Work out the finished part from the listing and answer in its coordinate system (mm). Coordinates: 2 decimals unless noted, no trailing zeros. Loops run counter-clockwise (first coordinate to the right, second up) from the corner with the lowest first, then second, coordinate; pieces in that order, holes last. Notation, with made-up numbers: (82, -27.75) -> (91, -27.75) arc R15 ccw to (91, -16.75) -> close; hole circle Ø1 at (-22, -8.75). An arc over 180 degrees is marked (long way). Use a Markdown table: item, result.
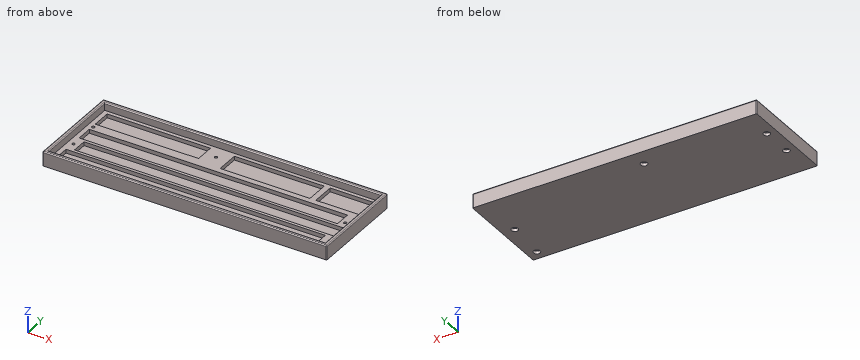
from build123d import *

# Parameters (mm, degrees)
SKETCH_W        = 297
SKETCH_H        = 102
PAD_DEPTH       = 15
SKETCH001_W     = 289
SKETCH001_H     = 94
POCKET_DEPTH    = 8
SKETCH002_W     = 271
SKETCH002_H     = 16
SKETCH002_W_2   = 272
SKETCH002_W_3   = 270
SKETCH002_H_2   = 17
SKETCH002_W_4   = 45.901761
SKETCH002_H_3   = 24
SKETCH002_W_5   = 94
SKETCH002_W_6   = 108
SKETCH002_H_4   = 20
POCKET001_DEPTH = 4
SKETCH003_R     = 1.51818
SKETCH003_R_2   = 1.523657
SKETCH003_R_3   = 1.522766
SKETCH003_R_4   = 1.49253
SKETCH003_R_5   = 1.485367
POCKET002_DEPTH = 15
SKETCH004_R     = 3.476644
SKETCH004_R_2   = 3.504577
SKETCH004_R_3   = 3.496918
SKETCH004_R_4   = 3.4664
SKETCH004_R_5   = 3.481812
POCKET003_DEPTH = 3
FILLET_R        = 1
FILLET001_R     = 1


with BuildPart() as part:
    # Sketch → Pad (new body)
    with BuildSketch(Plane.XY):
        with Locations((148.5, 51)):
            Rectangle(SKETCH_W, SKETCH_H)
    extrude(amount=PAD_DEPTH)

    # Sketch001 → Pocket (cut)
    with BuildSketch(Plane.XY.offset(15)):
        with Locations((148.5, 51)):
            Rectangle(SKETCH001_W, SKETCH001_H)
    extrude(amount=-POCKET_DEPTH, mode=Mode.SUBTRACT)

    # Sketch002 → Pocket001 (cut)
    with BuildSketch(Plane.XY.offset(7)):
        with Locations((144.5, 17)):
            Rectangle(SKETCH002_W, SKETCH002_H)
        with Locations((152, 36)):
            Rectangle(SKETCH002_W_2, SKETCH002_H)
        with Locations((144, 55.5)):
            Rectangle(SKETCH002_W_3, SKETCH002_H_2)
        with Locations((265.049119, 82)):
            Rectangle(SKETCH002_W_4, SKETCH002_H_3)
        with Locations((189, 82)):
            Rectangle(SKETCH002_W_5, SKETCH002_H_3)
        with Locations((63, 84)):
            Rectangle(SKETCH002_W_6, SKETCH002_H_4)
    extrude(amount=-POCKET001_DEPTH, mode=Mode.SUBTRACT)

    # Sketch003 → Pocket002 (cut)
    with BuildSketch(Plane.XY.offset(7)):
        with Locations((284, 52)):
            Circle(SKETCH003_R)
        with Locations((10, 36)):
            Circle(SKETCH003_R_2)
        with Locations((287, 10)):
            Circle(SKETCH003_R_3)
        with Locations((10, 69)):
            Circle(SKETCH003_R_4)
        with Locations((129, 84)):
            Circle(SKETCH003_R_5)
    extrude(amount=-POCKET002_DEPTH, mode=Mode.SUBTRACT)

    # Sketch004 → Pocket003 (cut)
    with BuildSketch(Plane(origin=(0, 0, 0), x_dir=(1, 0, 0), z_dir=(0, 0, -1))):
        with Locations((10, -36)):
            Circle(SKETCH004_R)
        with Locations((10, -69)):
            Circle(SKETCH004_R_2)
        with Locations((129, -84)):
            Circle(SKETCH004_R_3)
        with Locations((287, -10)):
            Circle(SKETCH004_R_4)
        with Locations((284, -52)):
            Circle(SKETCH004_R_5)
    extrude(amount=-POCKET003_DEPTH, mode=Mode.SUBTRACT)

    # Fillet
    fillet_edges = [part.edges().sort_by_distance(p)[0] for p in [
        (148.5, 102, 15),
        (297, 102, 7.5),
        (0, 102, 7.5),
        (148.5, 0, 15),
        (297, 0, 7.5),
        (0, 0, 7.5),
        (0, 51, 15),
        (297, 51, 15),
    ]]
    fillet(fillet_edges, radius=FILLET_R)

    # Fillet001
    fillet001_edges = [part.edges().sort_by_distance(p)[0] for p in [
        (148.5, 98, 15),
        (4, 51, 15),
        (148.5, 4, 15),
        (293, 51, 15),
    ]]
    fillet(fillet001_edges, radius=FILLET001_R)


solid = part.part
Q1. Section A-A on z = 11.5 is taken. Determine the outline of the cut face in (x, y), and give its area (3 significant figures).
Solved:
| item | result |
|---|---|
| outline | (0, 1) arc R1 ccw to (1, 0) -> (296, 0) arc R1 ccw to (297, 1) -> (297, 101) arc R1 ccw to (296, 102) -> (1, 102) arc R1 ccw to (0, 101) -> close; hole (4, 4) -> (293, 4) -> (293, 98) -> (4, 98) -> close |
| area | 3,130 mm² |
Q2. Section D-D on x = 95.5 is taken. Determine the outline of the cut face in (y, z), and give its area (3 significant figures).
Solved:
| item | result |
|---|---|
| outline | (0, 0) -> (102, 0) -> (102, 14) arc R1 ccw to (101, 15) -> (99, 15) arc R1 ccw to (98, 14) -> (98, 7) -> (94, 7) -> (94, 3) -> (74, 3) -> (74, 7) -> (64, 7) -> (64, 3) -> (47, 3) -> (47, 7) -> (44, 7) -> (44, 3) -> (28, 3) -> (28, 7) -> (25, 7) -> (25, 3) -> (9, 3) -> (9, 7) -> (4, 7) -> (4, 14) arc R1 ccw to (3, 15) -> (1, 15) arc R1 ccw to (0, 14) -> close |
| area | 501 mm² |
Q3. Section B-B on x = 201 is taken. Determine the outline of the cut face in (y, z), and give its area (3 significant figures).
Solved:
| item | result |
|---|---|
| outline | (0, 0) -> (102, 0) -> (102, 14) arc R1 ccw to (101, 15) -> (99, 15) arc R1 ccw to (98, 14) -> (98, 7) -> (94, 7) -> (94, 3) -> (70, 3) -> (70, 7) -> (64, 7) -> (64, 3) -> (47, 3) -> (47, 7) -> (44, 7) -> (44, 3) -> (28, 3) -> (28, 7) -> (25, 7) -> (25, 3) -> (9, 3) -> (9, 7) -> (4, 7) -> (4, 14) arc R1 ccw to (3, 15) -> (1, 15) arc R1 ccw to (0, 14) -> close |
| area | 485 mm² |
Q4. Given pin 1 Ø5 at (x, y) = (161.5, 51.5) entering from +Z; pin 2 Ø2.5 at (x, y) = (129, 84) entering from -Z; pin 3 Ø6.5 at (x, y) = (129, 84) entering from -Z; pin 4 Ø10 at (x, y) = (131.5, 29) entering from +Z, each flat-ended and moving along its own axis, determine where each tip first touches the part or whether it passes through.
Solved:
| item | result |
|---|---|
| pin 1 | z = 3 |
| pin 2 | through |
| pin 3 | z = 3 |
| pin 4 | z = 7 |
Q5. Consider line 1 (X direction, y = 91, z = 3.5); line 2 (Y direction, x = 152, z = 3.25); line 3 (Y direction, x = 10, z = 4.65). Determine where each line is inside the solid, lowest interval first. Write a range as [from, to].
Solved:
| item | result |
|---|---|
| line 1 | [0, 9], [117, 142], [236, 242.1], [288, 297] |
| line 2 | [0, 9], [25, 28], [44, 47], [64, 70], [94, 102] |
| line 3 | [0, 9], [25, 34.48], [37.52, 47], [64, 67.51], [70.49, 74], [94, 102] |
Q6. Section C-C on y = 17 is taken. Determine the outline of the cut face in (x, z), and give its area (3 significant figures).
Solved:
| item | result |
|---|---|
| outline | (0, 0) -> (297, 0) -> (297, 14) arc R1 ccw to (296, 15) -> (294, 15) arc R1 ccw to (293, 14) -> (293, 7) -> (280, 7) -> (280, 3) -> (9, 3) -> (9, 7) -> (4, 7) -> (4, 14) arc R1 ccw to (3, 15) -> (1, 15) arc R1 ccw to (0, 14) -> close |
| area | 1,060 mm² |
